Read the model definition and answer for the solid it produces. Units are mm, in the model's axes. A direction names the side the tool comes from. Round coordinates to 2 decimals unless told otherwise and drop trailing zeros. Order: outer loops, then holes, each group sorted by start corner. A loop starts at its lowest first (then second) coordinate and runs counter-clockwise, first axis right, second up. Notation, with made-up numbers: (-29.75, -36.75) - (-21.75, -36.75) arc R30 cw to (-21.75, -8.75) - close; hole circle Ø7 at (-19.75, 79). An arc over 180 degrees is marked (long way). Put each result on its own line as item: value. Start each with the question number.
Q1. Find the intervals of material crossed by line 1 along Y through (x, z) = (0, 1.15); line 2 along X through (y, z) = (1, 1.75); line 3 along X through (y, z) = (3, 10.5), in increasing order. Write a range as from..to.
Q2. Each of these flat-tipped pins is pushed along its axis until it touches: pin 1 Ø7 at (x, y) = (0, 0) entering from +Z; pin 2 Ø3 at (x, y) = (0, 0) entering from +Z; pin 3 Ø4 at (y, z) = (-2.5, 3) entering from +X; pin 4 Ø6 at (x, z) = (8.5, 9) entering from -Y. Where does it stop, or does it pass through?
Q3. Section A-A on x = 0 is taken. State how many separate pieces and enclosed holes the cut face has, then the cut area to 3 significant figures.
Q4. Section D-D on y = -4.5 is taken. Give the vertices of the cut face in (x, z).
Q5. Which of the six approach directions +Z, -Z, +X, -X, +Y, -Y give full straight-line access (tool end or side, diameter ignored) to faces 1 (the face through (-0.06, 7.14, 0.14)), 2 (the face through (-1.47, -6.64, 6.43))?
Q6. Section B-B on z = 6.5 is taken. Give the vertices of the cut face in (x, y).
Q7. Section C-C on x = 10 is taken. Give the vertices of the cut face in (y, z).
Q8. For a pull along X with two mould halves and no side action, classify faces 3 (the face through (7.5, 4.1, 1.2)), 4 (the face through (0, 2, 0.6)), 5 (the face through (-2.4, 0.1, 0)) as pulls with the +X half, pulls with the -X half, needs draft (parallel to the pull), parting line crosses it, or undercut.
from build123d import *

# Parameters (mm, degrees)
SKETCH_2_R          = 1.1
SKETCH_2_R_2        = 1
SKETCH_2_R_3        = 1.7
EXTRUDE_1_DEPTH     = 2
SKETCH_3_R          = 7.5
SKETCH_3_R_2        = 6.8
EXTRUDE_1_2_DEPTH   = 9.5
CUT_EXTRUDE_START   = -0.5
SKETCH_4_R          = 6.8
CUT_EXTRUDE_1_DEPTH = 0.5
SKETCH_5_R          = 2.25
CUT_EXTRUDE_2_DEPTH = 0.9
CHAMFER_1_SIZE      = 0.5


with BuildPart() as part:
    # Эскиз2 → Extrude 1 (new body)
    with BuildSketch(Plane.XY):
        with BuildLine():
            Line((4.05, 6.312487624), (11.134, 1.767496535))
            ThreePointArc((11.134, 1.767496535), (12.1, 0), (11.134, -1.767496535))
            Line((11.134, -1.767496535), (4.05, -6.312487624))
            ThreePointArc((4.05, -6.312487624), (0, -7.5), (-4.05, -6.312487624))
            Line((-4.05, -6.312487624), (-11.134, -1.767496535))
            ThreePointArc((-11.134, -1.767496535), (-12.1, 0), (-11.134, 1.767496535))
            Line((-11.134, 1.767496535), (-4.05, 6.312487624))
            ThreePointArc((-4.05, 6.312487624), (0, 7.5), (4.05, 6.312487624))
        make_face()
        with Locations((10, 0)):
            Circle(SKETCH_2_R, mode=Mode.SUBTRACT)
        with Locations((-10, 0)):
            Circle(SKETCH_2_R, mode=Mode.SUBTRACT)
        with Locations((0, 4.5)):
            Circle(SKETCH_2_R_2, mode=Mode.SUBTRACT)
        with Locations(Location((0, -4.5, 0), (0, 0, 180))):
            Circle(SKETCH_2_R_2, mode=Mode.SUBTRACT)
        Circle(SKETCH_2_R_3, mode=Mode.SUBTRACT)
    extrude(amount=EXTRUDE_1_DEPTH)

    # Эскиз3 → Extrude 1 2 (add)
    with BuildSketch(Plane.XY.offset(2)):
        Circle(SKETCH_3_R)
        Circle(SKETCH_3_R_2, mode=Mode.SUBTRACT)
    extrude(amount=EXTRUDE_1_2_DEPTH)

    # Эскиз4 → Вырез-Вытянуть1 (cut)
    with BuildSketch(Plane.XY.offset(2).offset(CUT_EXTRUDE_START)):
        Circle(SKETCH_4_R)
    extrude(amount=CUT_EXTRUDE_1_DEPTH, mode=Mode.SUBTRACT)

    # Эскиз5 → Вырез-Вытянуть2 (cut)
    with BuildSketch(Plane.XY.offset(1.5)):
        Circle(SKETCH_5_R)
    extrude(amount=-CUT_EXTRUDE_2_DEPTH, mode=Mode.SUBTRACT)

    # Фаска1
    chamfer_1_edges = [part.edges().sort_by_distance(p)[0] for p in [
        (-7.592, 4.039992079, 0),
        (0, 7.5, 0),
        (8.9, 0, 0),
        (-1, 4.5, 0),
        (1, -4.5, 0),
        (-1.7, 0, 0),
        (-11.1, 0, 0),
        (7.592, 4.039992079, 0),
        (12.1, 0, 0),
        (7.592, -4.039992079, 0),
        (0, -7.5, 0),
        (-7.592, -4.039992079, 0),
        (-12.1, 0, 0),
    ]]
    chamfer(chamfer_1_edges, length=CHAMFER_1_SIZE - 0.0001)  # a hair under: the kernel refuses the full size


solid = part.part
Findings:
1. line 1: -7.5..-5.5, -3.5..-2.25, 2.25..3.5, 5.5..7.5
1. line 2: -11.85..-10.46, -9.54..-6.73, 6.73..9.54, 10.46..11.85
1. line 3: -6.87..-6.1, 6.1..6.87
2. pin 1: z = 1.5
2. pin 2: through
2. pin 3: x = 11.95
2. pin 4: y = -5.1
3. separate pieces: 4
3. enclosed holes: 0
3. area: 23.4 mm2
4. outline: (-6.88, 0.5) - (-5.95, 0) - (-1.5, 0) - (-1, 0.5) - (-1, 1.5) - (-5.1, 1.5) - (-5.1, 11.5) - (-6, 11.5) - (-6, 2) - (-6.88, 2) - close; (1, 0.5) - (1.5, 0) - (5.95, 0) - (6.88, 0.5) - (6.88, 2) - (6, 2) - (6, 11.5) - (5.1, 11.5) - (5.1, 1.5) - (1, 1.5) - close
5. face 1: -Z, +Y
5. face 2: +Z
6. outline: circle Ø15 at (0, 0); hole circle Ø13.6 at (0, 0)
7. outline: (-2.5, 0.5) - (-1.9, 0) - (-1.6, 0) - (-1.1, 0.5) - (-1.1, 2) - (-2.5, 2) - close; (1.1, 0.5) - (1.6, 0) - (1.9, 0) - (2.5, 0.5) - (2.5, 2) - (1.1, 2) - close
8. face 3: pulls with the +X half
8. face 4: undercut
8. face 5: needs draft
